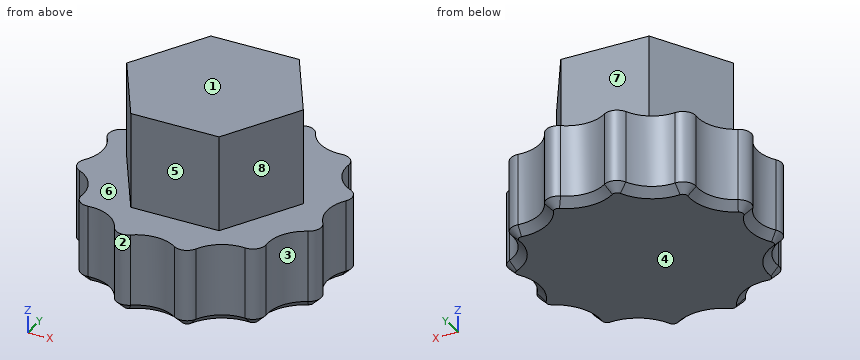
```python
from build123d import *

# Parameters (mm, degrees)
F1_DEPTH = 5
F3_DEPTH = 6
F4_SIZE  = 0.5


with BuildPart() as f1:
    # F0 (on Top) → F1 (new body)
    with BuildSketch(Plane.XY):
        with BuildLine():
            ThreePointArc((1.361869, 7.427878), (0, 7), (-1.361869, 7.427878))
            ThreePointArc((-1.361869, 7.427878), (-2.021263, 7.543457), (-2.534525, 7.113665))
            ThreePointArc((-2.534525, 7.113665), (-3.5, 6.062178), (-4.893352, 5.751796))
            ThreePointArc((-4.893352, 5.751796), (-5.522194, 5.522194), (-5.751796, 4.893352))
            ThreePointArc((-5.751796, 4.893352), (-6.062178, 3.5), (-7.113665, 2.534525))
            ThreePointArc((-7.113665, 2.534525), (-7.543457, 2.021263), (-7.427878, 1.361869))
            ThreePointArc((-7.427878, 1.361869), (-7, 0), (-7.427878, -1.361869))
            ThreePointArc((-7.427878, -1.361869), (-7.543457, -2.021263), (-7.113665, -2.534525))
            ThreePointArc((-7.113665, -2.534525), (-6.062178, -3.5), (-5.751796, -4.893352))
            ThreePointArc((-5.751796, -4.893352), (-5.522194, -5.522194), (-4.893352, -5.751796))
            ThreePointArc((-4.893352, -5.751796), (-3.5, -6.062178), (-2.534525, -7.113665))
            ThreePointArc((-2.534525, -7.113665), (-2.021263, -7.543457), (-1.361869, -7.427878))
            ThreePointArc((-1.361869, -7.427878), (0, -7), (1.361869, -7.427878))
            ThreePointArc((1.361869, -7.427878), (2.021263, -7.543457), (2.534525, -7.113665))
            ThreePointArc((2.534525, -7.113665), (3.5, -6.062178), (4.893352, -5.751796))
            ThreePointArc((4.893352, -5.751796), (5.522194, -5.522194), (5.751796, -4.893352))
            ThreePointArc((5.751796, -4.893352), (6.062178, -3.5), (7.113665, -2.534525))
            ThreePointArc((7.113665, -2.534525), (7.543457, -2.021263), (7.427878, -1.361869))
            ThreePointArc((7.427878, -1.361869), (7, 0), (7.427878, 1.361869))
            ThreePointArc((7.427878, 1.361869), (7.543457, 2.021263), (7.113665, 2.534525))
            ThreePointArc((7.113665, 2.534525), (6.062178, 3.5), (5.751796, 4.893352))
            ThreePointArc((5.751796, 4.893352), (5.522194, 5.522194), (4.893352, 5.751796))
            ThreePointArc((4.893352, 5.751796), (3.5, 6.062178), (2.534525, 7.113665))
            ThreePointArc((2.534525, 7.113665), (2.021263, 7.543457), (1.361869, 7.427878))
        make_face()
    extrude(amount=F1_DEPTH)

    # F2 (on face) → F3 (join)
    with BuildSketch(Plane.XY.offset(5)):
        Polygon((-2.749631, -4.7625), (2.749631, -4.7625), (5.499261, 0), (2.749631, 4.7625), (-2.749631, 4.7625), (-5.499261, 0), align=None)
    extrude(amount=F3_DEPTH)

    # F4
    f4_edges = [f1.edges().sort_by_distance(p)[0] for p in [
        (2.021263, 7.543457, 0),
        (0, 7, 0),
        (-2.021263, 7.543457, 0),
        (-3.5, 6.062178, 0),
        (-5.522194, 5.522194, 0),
        (-6.062178, 3.5, 0),
        (-7.543457, 2.021263, 0),
        (-7, 0, 0),
        (-7.543457, -2.021263, 0),
        (-6.062178, -3.5, 0),
        (-5.522194, -5.522194, 0),
        (-3.5, -6.062178, 0),
        (-2.021263, -7.543457, 0),
        (0, -7, 0),
        (2.021263, -7.543457, 0),
        (3.5, -6.062178, 0),
        (5.522194, -5.522194, 0),
        (6.062178, -3.5, 0),
        (7.543457, -2.021263, 0),
        (7, 0, 0),
        (7.543457, 2.021263, 0),
        (6.062178, 3.5, 0),
        (5.522194, 5.522194, 0),
        (3.5, 6.062178, 0),
    ]]
    chamfer(f4_edges, length=F4_SIZE)


solid = f1.part
```
Here's how the part is built. I have some questions about the finished solid (model axes, mm). Face numbers are marked on the shaded views. A direction names the side the tool comes from. Coordinates: 2 decimals unless noted, no trailing zeros. Order: outer loops, then holes, each group sorted by start corner. A loop starts at its lowest first (then second) coordinate and runs counter-clockwise, first axis right, second up.
1) Will these pins go through, and if not, where does the flat tip stop? pin 1 (6 mm diameter, centred on x = 0, z = 8.5, fed in from +Y); pin 2 (1 mm diameter, centred on x = 1.5, z = 8.5, fed in from -Y); pin 3 (3 mm diameter, centred on x = 6, z = 8, fed in from -Y).
2) Imagine slicing it at A-A on z = 6.25. List the corners of the cut face in (x, y) for me.
3) I need wall thicknesses on line 1 (Y direction, x = 1, z = 6.5); line 2 (X direction, y = 5, z = 3.75); line 3 (Y direction, x = 4.75, z = 3.25). Which ranges of each line are inside material? Lowest first, please.
4) Imagine slicing it at B-B on z = 2.5. List the corners of the cut face in (x, y) for me, and give its area (3 significant figures).
5) Which directions (+Z, -Z, +X, -X, +Y, -Y) give clear straight access to the entire face, cutting with the end or side of a thin tool? Please do the marked faces 4, 5, 6, 7 and 8.
6) We'd pull the mould along X, two halves only. Please class the marked faces 1, 2 and 3: +X half, -X half, draft (parallel to the pull), parting line (faces both ways), or undercut.
Response values:
1. pin 1: stops at y = 4.76
1. pin 2: stops at y = -4.76
1. pin 3: stops at y = -1.73
2. outline: (-5.5, 0) - (-2.75, -4.76) - (2.75, -4.76) - (5.5, 0) - (2.75, 4.76) - (-2.75, 4.76) - close
3. line 1: y = -4.76 to 4.76
3. line 2: x = -5.75 to 5.75
3. line 3: y = -5.74 to 5.74
4. outline: (-7.43, -1.36) arc R0.79 ccw to (-7.11, -2.53) arc R2.38 cw to (-5.75, -4.89) arc R0.79 ccw to (-4.89, -5.75) arc R2.38 cw to (-2.53, -7.11) arc R0.79 ccw to (-1.36, -7.43) arc R2.38 cw to (1.36, -7.43) arc R0.79 ccw to (2.53, -7.11) arc R2.38 cw to (4.89, -5.75) arc R0.79 ccw to (5.75, -4.89) arc R2.38 cw to (7.11, -2.53) arc R0.79 ccw to (7.43, -1.36) arc R2.38 cw to (7.43, 1.36) arc R0.79 ccw to (7.11, 2.53) arc R2.38 cw to (5.75, 4.89) arc R0.79 ccw to (4.89, 5.75) arc R2.38 cw to (2.53, 7.11) arc R0.79 ccw to (1.36, 7.43) arc R2.38 cw to (-1.36, 7.43) arc R0.79 ccw to (-2.53, 7.11) arc R2.38 cw to (-4.89, 5.75) arc R0.79 ccw to (-5.75, 4.89) arc R2.38 cw to (-7.11, 2.53) arc R0.79 ccw to (-7.43, 1.36) arc R2.38 cw to start
4. area: 170 mm2
5. face 4: -Z, +X, -X, +Y, -Y
5. face 5: +Z, +X, -X, -Y
5. face 6: +Z
5. face 7: +Z, +X, -X, +Y
5. face 8: +Z, +X, -Y
6. face 1: draft
6. face 2: undercut
6. face 3: +X half
